Autodesk Fusion 360 part; units mm, degrees
sketch "スケッチ1" plane through (0, 0, 0) normal (0, 0, 1) x (1, 0, 0)
  line L0 (333.3884, 190.0279) -> (333.3884, 8.0279)
  line L1 (337.8884, 190.0279) -> (337.8884, 8.0279)
  line L2 (342.3884, 3.5279) -> (383.3884, 3.5279)
  line L3 (342.3884, -0.9721) -> (383.3884, -0.9721)
  arc A0 (337.8884, 8.0279) -> (342.3884, 3.5279) centre (342.3884, 8.0279) ccw
  arc A1 (333.3884, 8.0279) -> (342.3884, -0.9721) centre (342.3884, 8.0279) ccw
  line L4 (383.3884, 3.5279) -> (383.3884, -0.9721)
  line L5 (342.3884, 199.0279) -> (383.3884, 199.0279)
  line L6 (342.3884, 194.5279) -> (383.3884, 194.5279)
  arc A2 (342.3884, 194.5279) -> (337.8884, 190.0279) centre (342.3884, 190.0279) ccw
  arc A3 (342.3884, 199.0279) -> (333.3884, 190.0279) centre (342.3884, 190.0279) ccw
  line L7 (383.3884, 199.0279) -> (383.3884, 194.5279)
  point P0 (333.3884, 199.0279)
extrude "押し出し1" add sketch "スケッチ1" along normal blind 100
Could you check a few things on this model? Use its own coordinates, in mm. A direction names the side the tool comes from. Give positions to 0.01 mm unless a question says otherwise; leave off trailing zeros. Order: outer loops, then holes, each group sorted by start corner. A loop starts at its lowest first (then second) coordinate and runs counter-clockwise, first axis right, second up.
Q1. I'm going to push flat-ended pins straight in: P1, Ø3, axis at y = 31, z = 44.5, coming from the +X side; P2, Ø4, axis at x = 341, y = 144, coming from the -Z side. Where does each tip first touch, or does it pass through?
Q2. Suppose I cut it at C-C, the plane y = 148.5. Write out the boundary of the cut face in (x, z).
Q3. Suppose I cut it at A-A, the plane x = 347.5. Write out the boundary of the cut face in (y, z), and give its area (3 significant figures).
Q4. We'd pull the mould along Y, two halves only. Please class faces 1 (the flat face through (336, 99, 0)), 2 (the flat face through (363, -0.972, 49)), 3 (the cylindrical face through (339.172, 193.175, 49.3)), 4 (the cylindrical face through (339.24, 4.81, 49.3)): +Y half, -Y half, draft (parallel to the pull), parting line (faces both ways), or undercut.
Q5. For faces 5 (the flat face through (333.388, 100, 49)), 6 (the flat face through (363, 3.528, 49)), which set-ups out of +Z, -Z, +X, -X, +Y, -Y let a thin tool reach every point of the face, with its end or its side?
Q6. If I drill on line 1 along Y through (x, z) = (381.5, 18.5); line 2 along X through (y, z) = (73.5, 81); line 3 along Y through (x, z) = (339, 59), over which ranges is the centre line in solid material (lowest first)?
Q7. Suppose I cut it at B-B, the plane z = 42.5. Write out the boundary of the cut face in (x, y).
Solution:
1. P1: stops at x = 337.89
1. P2: passes through
2. outline: (333.39, 0) - (337.89, 0) - (337.89, 100) - (333.39, 100) - close
3. outline: (-0.97, 0) - (3.53, 0) - (3.53, 100) - (-0.97, 100) - close; (194.53, 0) - (199.03, 0) - (199.03, 100) - (194.53, 100) - close
3. area: 900 mm2
4. face 1: draft
4. face 2: -Y half
4. face 3: undercut
4. face 4: undercut
5. face 5: +Z, -Z, -X, +Y, -Y
5. face 6: +Z, -Z, +X
6. line 1: y = -0.97 to 3.53, 194.53 to 199.03
6. line 2: x = 333.39 to 337.89
6. line 3: y = -0.31 to 5.07, 192.99 to 198.37
7. outline: (333.39, 8.03) arc R9 ccw to (342.39, -0.97) - (383.39, -0.97) - (383.39, 3.53) - (342.39, 3.53) arc R4.5 cw to (337.89, 8.03) - (337.89, 190.03) arc R4.5 cw to (342.39, 194.53) - (383.39, 194.53) - (383.39, 199.03) - (342.39, 199.03) arc R9 ccw to (333.39, 190.03) - close
